Design review of the part built by this model. Coordinates are the model's own, in mm. Face numbers are marked on the shaded views. A direction names the side the tool comes from. Round coordinates to 2 decimals unless told otherwise and drop trailing zeros. Loops run counter-clockwise (first coordinate to the right, second up) from the corner with the lowest first, then second, coordinate; pieces in that order, holes last. Notation, with made-up numbers: M 5,-24.5 L 56,-24.5 A10 ccw 56,-16.5 Z; hole C 12,75.25 d11. An arc over 180 degrees is marked long. One line per item, written item: value. Start each with the question number.
Item 1: We need section B-B (z = 2.1). Write out the cut boundary in (x, y), then the cut area to 3 significant figures.
Item 2: For the marked faces 1, 2 and 3, list the 3-axis set-ups (+Z, -Z, +X, -X, +Y, -Y) from which the entire face can be reached by the end or side of a thin tool; tool diameter is ignored.
Item 3: We need section D-D (x = -1.5). Write out the cut boundary in (y, z), then the cut area to 3 significant figures.
Item 4: Clearance check with flat-ended pins moving along their axes: pin 1 (0.5 mm diameter, centred on y = -2.5, z = 0.5, fed in from -X); pin 2 (1.5 mm diameter, centred on x = -5.5, y = -0.5, fed in from +Z); pin 3 (0.5 mm diameter, centred on y = 2.5, z = 0.5, fed in from +X); pin 4 (1 mm diameter, centred on x = -1.5, z = 2, fed in from -Y). State where each tip first meets the part, or that it passes through.
Item 5: Mouldability with a two-part tool opening along X and no side actions: class the marked faces 4, 5 and 6 as released by +X, released by -X, zero draft, split by the parting line, or undercut.
Item 6: For line 1 along Z through (x, y) = (1, 0); line 2 along X through (y, z) = (1.75, 1.55); line 3 along X through (y, z) = (-1.25, 2.5), list the stretches that pass through material, from the lowest coordinate up.
Item 7: We need section C-C (z = 0.5). Write out the cut boundary in (x, y), then the cut area to 3 significant figures.
Item 8: We need section A-A (y = 1.75). Write out the cut boundary in (x, z), then the cut area to 3 significant figures.
Autodesk Inventor part; units mm, degrees
ref_plane "YZ Plane" through (0, 0, 0) normal (1, 0, 0) x (0, 1, 0)
ref_plane "XZ Plane" through (0, 0, 0) normal (0, 1, 0) x (-1, 0, 0)
ref_plane "XY Plane" through (0, 0, 0) normal (0, 0, 1) x (1, 0, 0)
sketch "Boceto1" plane through (0, 0, 0) normal (0, 1, 0) x (-1, 0, 0)
  arc A0 (0, 0) -> (4.0155, 1.6275) centre (-0.0005, 5.7684) ccw
  arc A1 (0, 0.9884) -> (3.6027, 2.6275) centre (-0.0005, 5.7684) ccw
  line L0 (4.0155, 1.6275) -> (5.0155, 1.6275)
  line L1 (6.0155, 1.6275) -> (6.5155, 1.6275)
  line L2 (6.5155, 1.6275) -> (6.5155, 2.6275)
  line L3 (6.5155, 2.6275) -> (3.6027, 2.6275)
  line L4 (0, 0.9884) -> (0, 0)
  arc A2 (-4.0155, 1.6275) -> (0, 0) centre (0.0005, 5.7684) ccw
  arc A3 (-4.0892, 3.294) -> (0, 0.9884) centre (0.0005, 5.7684) ccw
  line L5 (-4.0155, 1.6275) -> (-4.5782, 0.8009)
  line L6 (-4.5782, 0.8009) -> (-5.4045, 1.3641)
  line L7 (-5.4045, 1.3641) -> (-4.0892, 3.294)
  line L8 (5.0155, 1.6275) -> (6.0155, 1.6275)
  dimension "d1" = 4.78
  dimension "d2" = 1
  dimension "d3" = 1
  dimension "d4" = 0.5
  dimension "d5" = 1
  dimension "d6" = 1
  dimension "d7" = 1
extrude "Extrusión1" add sketch "Boceto1" along normal mid plane 6
sketch "Boceto2" plane through (-4.0155, 3, 1.6275) normal (0, 0, -1) x (-1, 0, 0)
  line L0 (2.5, -6) -> (2.5, 0)
  line L1 (0, 0) -> (2.5, 0)
  line L2 (0, -6) -> (0, 0)
  line L3 (2.5, -6) -> (0, -6)
  circle A0 centre (1.25, -3) radius 0.8
  line L4 (1.25, -2.2) -> (1.25, -3.8)
  point P0 (-4.0155, -3)
  dimension "d10" = 1.6
revolve "Revolución1" add sketch "Boceto2" angle 360 about axis through (-5.2655, 0.8, 1.6275) along (0, -1, 0) picked at (1.0732, -3.1996) contours L4 A0
ref_plane "Plano de trabajo1" through (0.9621, 4, -0.4105) normal (0, 1, 0) x (1, 0, 0)
sketch "Boceto3" plane through (0.9621, 4, -0.4105) normal (0, 1, 0) x (1, 0, 0)
  line L0 (0.027, -3.311) -> (-1.1061, -3.311)
  line L1 (-1.1061, -3.311) -> (-1.1061, 0.0355)
  line L2 (-1.1061, 0.0355) -> (0.027, 0.0355)
  line L3 (0.027, 0.0355) -> (0.027, -3.311)
  point P0 (-0.9621, -0.4105)
  dimension "d14" = 3.3465
extrude "Extrusión2" cut sketch "Boceto3" against normal blind 2
ref_plane "Plano de trabajo2" through (0, 0, 0) normal (0, 1, 0) x (1, 0, 0)
mirror "Simetría1" about plane through (0, 0, 0) normal (0, 1, 0) of "Extrusión2"
fillet "Empalme1" radius 0.7 4 edges at (-6.5155, 3, 2.1275) (-6.5155, -3, 2.1275) (4.9914, -3, 1.0825) (4.9914, 3, 1.0825)
fillet "Empalme2" radius 0.3 1 edges at (4.0892, 0, 3.294)
fillet "Empalme3" radius 0.3 1 edges at (4.0155, 0, 1.6275)
properties part number "InteriorSw" material "----------"
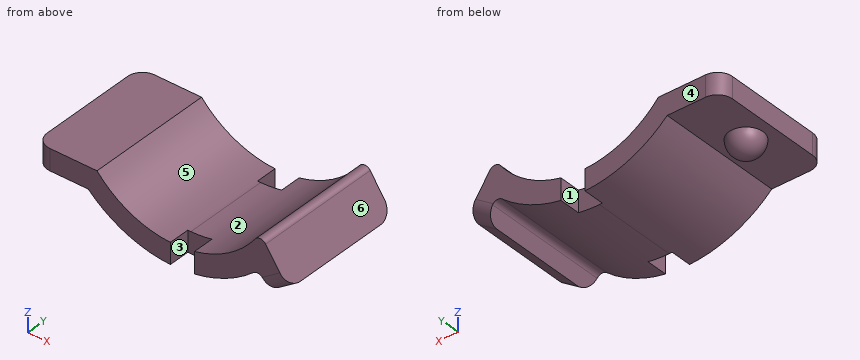
A:
1. outline: M -6.52,-2.3 A0.7 ccw -5.82,-3 L -3.06,-3 L -3.06,3 L -5.82,3 A0.7 ccw -6.52,2.3 Z; M 3.06,-3 L 4.9,-3 L 4.9,3 L 3.06,3 Z
1. area: 31.5 mm2
2. face 1: +Z, -Z, +Y
2. face 2: +Z, +Y, -Y
2. face 3: +Z, -Z, -Y
3. outline: M -3,0.2 L 3,0.2 L 3,1.23 L -3,1.23 Z
3. area: 6.19 mm2
4. pin 1: x = -2.84
4. pin 2: z = 2.63
4. pin 3: x = 2.84
4. pin 4: through
5. face 4: zero draft
5. face 5: undercut
5. face 6: released by +X
6. line 1: 0.09 to 1.09
6. line 2: -3.93 to -2.25, 2.25 to 5.28
6. line 3: -6.52 to -3.49, 3.49 to 4.63
7. outline: M -2.35,-3 L -0.14,-3 L -0.14,-2 L 0.99,-2 L 0.99,-3 L 2.35,-3 L 2.35,3 L 0.99,3 L 0.99,2 L -0.14,2 L -0.14,3 L -2.35,3 Z
7. area: 25.9 mm2
8. outline: M -6.52,1.63 L -4.02,1.63 A5.77 ccw 0,0 A5.77 ccw 3.77,1.4 A0.3 cw 4.21,1.34 L 4.58,0.8 L 5.4,1.36 L 4.34,2.93 A0.3 ccw 3.85,2.94 A4.78 cw 0,0.99 A4.78 cw -3.6,2.63 L -6.52,2.63 Z
8. area: 13.1 mm2
